from build123d import *

# Parameters (mm, degrees)
SKETCH1_R             = 3.75
SKETCH1_R_2           = 1.75
BOSS_EXTRUDE1_DEPTH   = 10
BOSS_EXTRUDE1_2_DEPTH = 10
BOSS_EXTRUDE2_START   = -3
BOSS_EXTRUDE2_DEPTH   = 3
SKETCH3_R             = 2.5
CUT_EXTRUDE1_DEPTH    = 57.367102098
CUT_EXTRUDE2_DEPTH    = 57.367102098


with BuildPart() as part:
    # Sketch1 → Boss-Extrude1 (new body)
    with BuildSketch(Plane.XZ.offset(100.2)):
        with Locations(Location((-39.876255843, 0, 0), (0, 0, 270))):
            Circle(SKETCH1_R)
        with Locations(Location((-39.876255843, 0, 0), (0, 0, 270))):
            Circle(SKETCH1_R_2, mode=Mode.SUBTRACT)
    extrude(amount=BOSS_EXTRUDE1_DEPTH)



with BuildPart() as body_2:
    # Sketch1 → Boss-Extrude1 2 (new body)
    with BuildSketch(Plane.XZ.offset(100.2)):
        with Locations(Location((39.876255843, 0, 0), (0, 0, 90))):
            Circle(SKETCH1_R)
        with Locations(Location((39.876255843, 0, 0), (0, 0, 90))):
            Circle(SKETCH1_R_2, mode=Mode.SUBTRACT)
    extrude(amount=BOSS_EXTRUDE1_2_DEPTH)


with BuildPart() as part_1:
    add(part.part)

    add(body_2.part)  # Boss-Extrude2 merges body 2
    # Sketch2 → Boss-Extrude2 (add)
    with BuildSketch(Plane.XZ.offset(110.2).offset(BOSS_EXTRUDE2_START)):
        with BuildLine():
            Line((25, 35), (-25, 35))
            Line((-25, 35), (-43.165990296, 1.800040897))
            ThreePointArc((-43.165990296, 1.800040897), (-38.94727904, 3.633111903), (-36.126255843, 0))
            ThreePointArc((-36.126255843, 0), (-38.94727904, -3.633111903), (-43.165990296, -1.800040897))
            Line((-43.165990296, -1.800040897), (-25, -35))
            Line((-25, -35), (25, -35))
            Line((25, -35), (43.165990296, -1.800040897))
            ThreePointArc((43.165990296, -1.800040897), (36.126255843, 0), (43.165990296, 1.800040897))
            Line((43.165990296, 1.800040897), (25, 35))
        make_face()
        with BuildLine():
            Line((-25, 19.375354996), (-25, -19.375354996))
            Line((-25, -19.375354996), (-32.975123568, -4.800109057))
            ThreePointArc((-32.975123568, -4.800109057), (-34.20249836, 0), (-32.975123568, 4.800109057))
            Line((-32.975123568, 4.800109057), (-25, 19.375354996))
        make_face(mode=Mode.SUBTRACT)
        with BuildLine():
            Line((32.975123568, -4.800109057), (25, -19.375354996))
            Line((25, -19.375354996), (25, 19.375354996))
            Line((25, 19.375354996), (32.975123568, 4.800109057))
            ThreePointArc((32.975123568, 4.800109057), (34.20249836, 0), (32.975123568, -4.800109057))
        make_face(mode=Mode.SUBTRACT)
    extrude(amount=BOSS_EXTRUDE2_DEPTH)

    # Sketch3 → Cut-Extrude1 (cut, through all)
    with BuildSketch(Plane(origin=(0, -107.2, 0), x_dir=(1, 0, 0), z_dir=(0, 1, 0))):
        with Locations(Location((0, 0, 0), (0, 0, 270))):
            Circle(SKETCH3_R)
    extrude(amount=-CUT_EXTRUDE1_DEPTH, mode=Mode.SUBTRACT)

    # Sketch4 → Cut-Extrude2 (cut, through all)
    with BuildSketch(Plane(origin=(0, -107.2, 0), x_dir=(1, 0, 0), z_dir=(0, 1, 0))):
        with BuildLine():
            Line((20, -17.807929785), (-20, -17.807929785))
            ThreePointArc((-20, -17.807929785), (-21.25, -19.057929785), (-20, -20.307929785))
            Line((-20, -20.307929785), (20, -20.307929785))
            ThreePointArc((20, -20.307929785), (21.25, -19.057929785), (20, -17.807929785))
        make_face()
        with BuildLine():
            Line((20, 20.307929785), (-20, 20.307929785))
            ThreePointArc((-20, 20.307929785), (-21.25, 19.057929785), (-20, 17.807929785))
            Line((-20, 17.807929785), (20, 17.807929785))
            ThreePointArc((20, 17.807929785), (21.25, 19.057929785), (20, 20.307929785))
        make_face()
    extrude(amount=-CUT_EXTRUDE2_DEPTH, mode=Mode.SUBTRACT)


solid = part_1.part
Work out the finished part from the listing and answer in its coordinate system (mm). A direction names the side the tool comes from. Round coordinates to 2 decimals unless told otherwise and drop trailing zeros. Loops run counter-clockwise (first coordinate to the right, second up) from the corner with the lowest first, then second, coordinate; pieces in that order, holes last. Notation, with made-up numbers: (59, 33) - (70, 33) arc R18 ccw to (70, 68) - close; hole circle Ø3 at (-11.5, 72). An arc over 180 degrees is marked (long way). Use one line per item in the form item = value. Start each with the question number.
(1) Flat-ended cylindrical pins translate along their axes: P1, Ø1.5, axis at x = 18, y = -105.5, coming from the -Z side; P2, Ø10, axis at x = 4, z = -22, coming from the +Y side; P3, Ø3.5, axis at y = -108.5, z = 7, coming from the -X side; P4, Ø3.5, axis at y = -109, z = 5.5, coming from the +X side. Find the tip coordinate at first contact, or state that the pin passes through.
(2) Determine the mould class of faces 4 (the face through (-33.956, -108.679, 18.632)), 5 (the face through (21.25, -108.68, 19.09)), 6 (the face through (-43.203, -104.019, -1.73)), 7 (the face through (-1, -110.2, 8)) for opening direction Z: +Z half, -Z half, draft (parallel to the pull), parting line (faces both ways), or undercut.
(3) Find section C-C on z = -16. Determine the outline of the cut face in (x, y).
(4) Find section B-B on z = 0. Determine the outline of the cut face in (x, y), and give its area (3 significant figures).
(5) Find section A-A on x = 0. Determine the outline of the cut face in (y, z), and give its area (3 significant figures).
(6) Which of the six approach directions +Z, -Z, +X, -X, +Y, -Y give full straight-line access (tool end or side, diameter ignored) to faces 1 (the face through (43.203, -104.019, 1.73)), 2 (the face through (0, -109, 35)), 3 (the face through (-21.25, -108.68, 19.03))?
(7) Find section D-D on y = -104.25. Determine the outline of the cut face in (x, z), and give its area (3 significant figures).
(8) Consider line 1 (Z direction, x = 11, y = -108.5); line 2 (X direction, y = -106.25, z = 0); line 3 (X direction, y = -109.5, z = 14.5). Determine where each line is inside the solid, lowest interval first.
Answer list:
q1.P1 = through
q1.P2 = -107.2
q1.P3 = -41.28
q1.P4 = 42.1
q2.face_4 = +Z half
q2.face_5 = undercut
q2.face_6 = parting line
q2.face_7 = draft
q3.outline = (-35.4, -110.2) - (-26.85, -110.2) - (-26.85, -107.2) - (-35.4, -107.2) - close; (-25, -110.2) - (25, -110.2) - (25, -107.2) - (-25, -107.2) - close; (26.85, -110.2) - (35.4, -110.2) - (35.4, -107.2) - (26.85, -107.2) - close
q4.outline = (-43.63, -110.2) - (-41.63, -110.2) - (-41.63, -100.2) - (-43.63, -100.2) - close; (-38.13, -110.2) - (-34.2, -110.2) - (-34.2, -107.2) - (-36.13, -107.2) - (-36.13, -100.2) - (-38.13, -100.2) - close; (-25, -110.2) - (-2.5, -110.2) - (-2.5, -107.2) - (-25, -107.2) - close; (2.5, -110.2) - (25, -110.2) - (25, -107.2) - (2.5, -107.2) - close; (34.2, -110.2) - (38.13, -110.2) - (38.13, -100.2) - (36.13, -100.2) - (36.13, -107.2) - (34.2, -107.2) - close; (41.63, -110.2) - (43.63, -110.2) - (43.63, -100.2) - (41.63, -100.2) - close
q4.area = 227 mm^2
q5.outline = (-110.2, -35) - (-107.2, -35) - (-107.2, -20.31) - (-110.2, -20.31) - close; (-110.2, -17.81) - (-107.2, -17.81) - (-107.2, -2.5) - (-110.2, -2.5) - close; (-110.2, 2.5) - (-107.2, 2.5) - (-107.2, 17.81) - (-110.2, 17.81) - close; (-110.2, 20.31) - (-107.2, 20.31) - (-107.2, 35) - (-110.2, 35) - close
q5.area = 180 mm^2
q6.face_1 = +Y
q6.face_2 = +Z, +X, -X, +Y, -Y
q6.face_3 = +Y, -Y
q7.outline = circle Ø7.5 at (-39.88, 0); circle Ø7.5 at (39.88, 0); hole circle Ø3.5 at (-39.88, 0); hole circle Ø3.5 at (39.88, 0)
q7.area = 69.1 mm^2
q8.line_1 = -35 to -20.31, -17.81 to 17.81, 20.31 to 35
q8.line_2 = -43.63 to -41.63, -38.13 to -36.13, 36.13 to 38.13, 41.63 to 43.63
q8.line_3 = -36.22 to -27.67, -25 to 25, 27.67 to 36.22
